The model under review builds one solid part; all positions refer to its coordinate system, in mm. A direction names the side the tool comes from. Give positions to 0.01 mm unless a question says otherwise; leave off trailing zeros. Loops run counter-clockwise (first coordinate to the right, second up) from the corner with the lowest first, then second, coordinate; pieces in that order, holes last. Notation, with made-up numbers: (41, 75.5) - (71, 75.5) arc R21 ccw to (71, 103.5) - close; hole circle Ø4 at (-7, -9). An arc over 180 degrees is marked (long way). Return JSON: item names as keys, results as strings. Group by question number.
from build123d import *

# Parameters (mm, degrees)
SKETCH2_W           = 12.5
SKETCH2_H           = 13.4
BOSS_EXTRUDE1_DEPTH = 7.5
SKETCH3_R           = 3.05
BOSS_EXTRUDE2_DEPTH = 20
SKETCH4_W           = 20
SKETCH4_H           = 20
BOSS_EXTRUDE3_DEPTH = 2


with BuildPart() as part:
    # Sketch2 → Boss-Extrude1 (new body)
    with BuildSketch(Plane(origin=(0, 0, 0), x_dir=(1, 0, 0), z_dir=(0, 1, 0))):
        Rectangle(SKETCH2_W, SKETCH2_H)
    extrude(amount=BOSS_EXTRUDE1_DEPTH)

    # Sketch3 → Boss-Extrude2 (add)
    with BuildSketch(Plane(origin=(0, 7.5, 0), x_dir=(1, 0, 0), z_dir=(0, 1, 0))):
        with Locations(Location((0, 0, 0), (0, 0, 270))):
            Circle(SKETCH3_R)
    extrude(amount=BOSS_EXTRUDE2_DEPTH)

    # Sketch4 → Boss-Extrude3 (add)
    with BuildSketch(Plane.XZ):
        with Locations((0, -1.9)):
            Rectangle(SKETCH4_W, SKETCH4_H)
    extrude(amount=BOSS_EXTRUDE3_DEPTH)


solid = part.part
Item 1: Tool access review of faces 1 (the face through (6.25, 4, 0)), 2 (the face through (-6.25, 4, 0)), 3 (the face through (-3, 7.5, -2)): name each direction out of +Z, -Z, +X, -X, +Y, -Y from which nothing blocks a thin tool from reaching the whole face with its end or side.
Item 2: Take a section at A-A (x = -5.75). State the section outline as (y, z) points, then the cut area to 4 significant figures.
Item 3: Mouldability with a two-part tool opening along Z and no side actions: class faces 4 (the face through (10, -1, -2)), 5 (the face through (0, 4, -6.7)), 6 (the face through (0, -1, 8.1)), 7 (the face through (-1.856, 17.36, -2.42)) as +Z half, -Z half, draft (parallel to the pull), parting line (faces both ways), or undercut.
Item 4: Take a section at D-D (x = -1.5). State the section outline as (y, z) points, then the cut area to 3 significant figures.
Item 5: Take a section at C-C (y = 3). State the section outline as (x, z) points, then the cut area to 4 significant figures.
Item 6: For L1, parallel to Z at x = 3.25, y = 2; L2, parallel to Y at x = 8.25, z = 4; L3, parallel to Y at x = 3.5, z = -0.5, list the stretches that pass through material, from the lowest coordinate up. Write a range as from..to.
Item 7: For P1, Ø8, axis at x = 2, z = -2.5, coming from the +Y side; P2, Ø5, axis at x = 2.5, y = 17.5, coming from the +Z side; P3, Ø2, axis at y = 3, z = -3.5, coming from the +X side; P4, Ø1.5, axis at x = 4, y = 11.5, coming from the +Z side, all flat-tipped, find the tip position at first contact; note any pin that passes through.
Item 8: Take a section at B-B (z = 0). State the section outline as (x, y) points.
Check sheet entries:
{
 "1": {"face 1": "+Z, -Z, +X, +Y", "face 2": "+Z, -Z, -X, +Y", "face 3": "+Y"},
 "2": {"outline": "(-2, -11.9) - (0, -11.9) - (0, -6.7) - (7.5, -6.7) - (7.5, 6.7) - (0, 6.7) - (0, 8.1) - (-2, 8.1) - close", "area": "140.5 mm^2"},
 "3": {"face 4": "draft", "face 5": "-Z half", "face 6": "+Z half", "face 7": "parting line"},
 "4": {"outline": "(-2, -11.9) - (0, -11.9) - (0, -6.7) - (7.5, -6.7) - (7.5, -2.66) - (27.5, -2.66) - (27.5, 2.66) - (7.5, 2.66) - (7.5, 6.7) - (0, 6.7) - (0, 8.1) - (-2, 8.1) - close", "area": "247 mm^2"},
 "5": {"outline": "(-6.25, -6.7) - (6.25, -6.7) - (6.25, 6.7) - (-6.25, 6.7) - close", "area": "167.5 mm^2"},
 "6": {"L1": "z = -6.7..6.7", "L2": "y = -2..0", "L3": "y = -2..7.5"},
 "7": {"P1": "stops at y = 27.5", "P2": "stops at z = 3.05", "P3": "stops at x = 6.25", "P4": "passes through"},
 "8": {"outline": "(-10, -2) - (10, -2) - (10, 0) - (6.25, 0) - (6.25, 7.5) - (3.05, 7.5) - (3.05, 27.5) - (-3.05, 27.5) - (-3.05, 7.5) - (-6.25, 7.5) - (-6.25, 0) - (-10, 0) - close"}
}
